Build history of the part. All positions in model axes, mm. Face numbers are marked on the shaded views. A direction names the side the tool comes from. Round coordinates to 2 decimals unless told otherwise and drop trailing zeros. Write each loop counter-clockwise with the first axis right and the second up, starting at its lowest first coordinate (ties: lowest second). Pieces come first, ordered by that corner, then holes. Notation, with made-up numbers: (88, -33) - (99, -33) arc R24 cw to (99, -5) - close; hole circle Ø10 at (17.25, -12.75). An arc over 180 degrees is marked (long way). Write each question's results on one line, items separated by ' | '.
from build123d import *

# Parameters (mm, degrees)
F0_W      = 14
F0_H      = 14
F1_DEPTH  = 7
F2_R      = 2.5
F4_DEPTH  = 2
F5_SIZE   = 2.99999
F6_R      = 2.5
F11_DEPTH = 2
F7_R      = 2.5
F12_DEPTH = 2
F8_R      = 2.5
F13_DEPTH = 2
F9_R      = 2.5
F14_DEPTH = 2
F10_R     = 2.5
F15_DEPTH = 2


# Not quite as in the source:
# - a fillet or chamfer is up to 0.001 mm smaller than in the source, because OpenCascade refuses the exact size


with BuildPart() as f1:
    # F0 (on Top) → F1 (new body, symmetric)
    with BuildSketch(Plane.XY):
        Rectangle(F0_W, F0_H)
    extrude(amount=F1_DEPTH, both=True)

    # F2 (on face) → F4 (cut)
    with BuildSketch(Plane.YZ.offset(7)):
        Polygon((-4, 1.6568542495), (-4, -1.6568542495), (-1.6568542495, -4), (1.6568542495, -4), (4, -1.6568542495), (4, 1.6568542495), (1.6568542495, 4), (-1.6568542495, 4), align=None)
        Circle(F2_R, mode=Mode.SUBTRACT)
    extrude(amount=-F4_DEPTH, mode=Mode.SUBTRACT)

    # F5 (size 3 in the source; OpenCascade refuses exactly that, so slightly less here)
    f5_edges = [f1.edges().sort_by_distance(p)[0] for p in [
        (7, 7, 0),
        (0, 7, -7),
        (-7, 7, 0),
        (0, 7, 7),
        (0, -7, 7),
        (7, 0, 7),
        (-7, 0, 7),
        (0, -7, -7),
        (7, -7, 0),
        (-7, -7, 0),
        (7, 0, -7),
        (-7, 0, -7),
    ]]
    chamfer(f5_edges, length=F5_SIZE)

    # F6 (on face) → F11 (cut)
    with BuildSketch(Plane(origin=(0, 7, 0), x_dir=(-1, 0, 0), z_dir=(0, 1, 0))):
        Polygon((-4, 1.6568542495), (-4, -1.6568542495), (-1.6568542495, -4), (1.6568542495, -4), (4, -1.6568542495), (4, 1.6568542495), (1.6568542495, 4), (-1.6568542495, 4), align=None)
        Circle(F6_R, mode=Mode.SUBTRACT)
    extrude(amount=-F11_DEPTH, mode=Mode.SUBTRACT)

    # F7 (on face) → F12 (cut)
    with BuildSketch(Plane.XY.offset(7)):
        Polygon((-4, 1.6568542495), (-4, -1.6568542495), (-1.6568542495, -4), (1.6568542495, -4), (4, -1.6568542495), (4, 1.6568542495), (1.6568542495, 4), (-1.6568542495, 4), align=None)
        Circle(F7_R, mode=Mode.SUBTRACT)
    extrude(amount=-F12_DEPTH, mode=Mode.SUBTRACT)

    # F8 (on face) → F13 (cut)
    with BuildSketch(Plane(origin=(-7, 0, 0), x_dir=(0, -1, 0), z_dir=(-1, 0, 0))):
        Polygon((-4, 1.6568542495), (-4, -1.6568542495), (-1.6568542495, -4), (1.6568542495, -4), (4, -1.6568542495), (4, 1.6568542495), (1.6568542495, 4), (-1.6568542495, 4), align=None)
        Circle(F8_R, mode=Mode.SUBTRACT)
    extrude(amount=-F13_DEPTH, mode=Mode.SUBTRACT)

    # F9 (on face) → F14 (cut)
    with BuildSketch(Plane.XZ.offset(7)):
        Polygon((-4, 1.6568542495), (-4, -1.6568542495), (-1.6568542495, -4), (1.6568542495, -4), (4, -1.6568542495), (4, 1.6568542495), (1.6568542495, 4), (-1.6568542495, 4), align=None)
        Circle(F9_R, mode=Mode.SUBTRACT)
    extrude(amount=-F14_DEPTH, mode=Mode.SUBTRACT)

    # F10 (on face) → F15 (cut)
    with BuildSketch(Plane(origin=(0, 0, -7), x_dir=(1, 0, 0), z_dir=(0, 0, -1))):
        Polygon((-4, 1.6568542495), (-4, -1.6568542495), (-1.6568542495, -4), (1.6568542495, -4), (4, -1.6568542495), (4, 1.6568542495), (1.6568542495, 4), (-1.6568542495, 4), align=None)
        Circle(F10_R, mode=Mode.SUBTRACT)
    extrude(amount=-F15_DEPTH, mode=Mode.SUBTRACT)


solid = f1.part
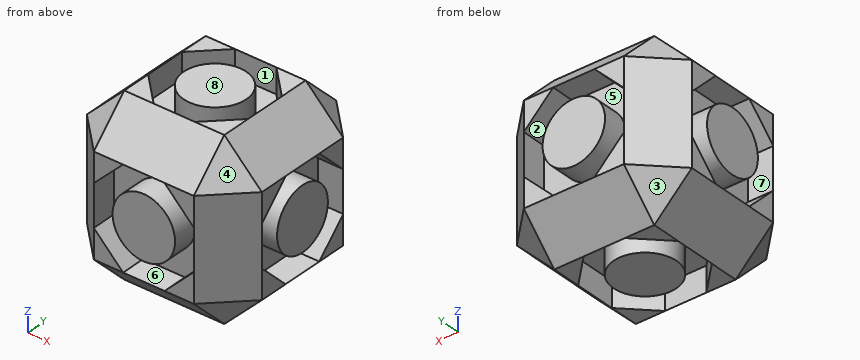
(1) Slice it at A-A, the plane z = 5.25. Write the cut outline in (x, y), and give its area (3 significant figures).
Worked answers:
outline: (-5.75, -4) - (-4, -5.75) - (4, -5.75) - (5.75, -4) - (5.75, 4) - (4, 5.75) - (-4, 5.75) - (-5.75, 4) - close; circle Ø5 at (0, 0); hole (-4, -1.66) - (-1.66, -4) - (1.66, -4) - (4, -1.66) - (4, 1.66) - (1.66, 4) - (-1.66, 4) - (-4, 1.66) - close | area: 92.7 mm2
(2) Drill centre lines: probe 1 along X at (y, z) = (5.75, 2); probe 2 along Z at (x, y) = (-6, -1.5); probe 3 along Z at (x, y) = (-1.75, -5.5). Where is each one in solid material? Low to high. Write a range as [from, to].
Worked answers:
probe 1: x = [-5.25, -3.66], [-1.5, 1.5], [3.66, 5.25] | probe 2: z = [-5, -4], [-2, 2], [4, 5] | probe 3: z = [-5.5, -3.91], [-1.79, 1.79], [3.91, 5.5]
(3) Flat gauge pins, fed straight in: pin 1 Ø0.6 at (x, y) = (0, -6.5) entering from +Z; pin 2 Ø2 at (x, y) = (-6, 0) entering from +Z; pin 3 Ø2 at (x, z) = (6, 0) entering from +Y. Where does each tip first touch, or does it go through?
Worked answers:
pin 1: stops at z = 4.8 | pin 2: stops at z = 6 | pin 3: stops at y = 6
(4) Tool access for the marked faces 5, 6, 7 and 8: list every direction of +Z, -Z, +X, -X, +Y, -Y with a clear straight run to the whole face (end or side of a thin tool).
Worked answers:
face 5: +Y | face 6: -Y | face 7: -X | face 8: +Z, +X, -X, +Y, -Y
(5) Slice it at C-C, the plane y = -4.25. Write the cut outline in (x, z).
Worked answers:
outline: (-6.75, -4) - (-4, -6.75) - (4, -6.75) - (6.75, -4) - (6.75, 4) - (4, 6.75) - (-4, 6.75) - (-6.75, 4) - close
(6) Slice it at B-B, the plane x = 6. Write the cut outline in (y, z), and give its area (3 significant figures).
Worked answers:
outline: (-5, -4) - (-4, -5) - (4, -5) - (5, -4) - (5, 4) - (4, 5) - (-4, 5) - (-5, 4) - close; circle Ø5 at (0, 0); hole (-4, -1.66) - (-1.66, -4) - (1.66, -4) - (4, -1.66) - (4, 1.66) - (1.66, 4) - (-1.66, 4) - (-4, 1.66) - close | area: 64.6 mm2
(7) Two-plate mould, pull along X, no slides. Class the marked faces 1, 2, 3 and 4: released by +X, released by -X, zero draft, split by the parting line, or undercut.
Worked answers:
face 1: undercut | face 2: undercut | face 3: released by -X | face 4: released by +X
(8) Slice it at D-D, the plane y = 3.75. Write the cut outline in (x, z).
Worked answers:
outline: (-7, -4) - (-4, -7) - (-1.91, -7) - (-1.91, -5) - (1.91, -5) - (1.91, -7) - (4, -7) - (7, -4) - (7, -1.91) - (5, -1.91) - (5, 1.91) - (7, 1.91) - (7, 4) - (4, 7) - (1.91, 7) - (1.91, 5) - (-1.91, 5) - (-1.91, 7) - (-4, 7) - (-7, 4) - (-7, 1.91) - (-5, 1.91) - (-5, -1.91) - (-7, -1.91) - close
